Work out the finished part from the listing and answer in its coordinate system (mm). Round coordinates to 2 decimals unless told otherwise and drop trailing zeros. Order: outer loops, then holes, each group sorted by start corner. A loop starts at its lowest first (then second) coordinate and runs counter-clockwise, first axis right, second up. Notation, with made-up numbers: (-19, 56.25) -> (23, 56.25) arc R15 ccw to (23, 83.25) -> close; hole circle Ø3 at (83.25, -32). An arc over 180 degrees is marked (long way). Use a Markdown table: item, result. Add a question column.
Item 1: A cutting plane is placed at A-A, the plane z = 869. Determine the outline of the cut face in (x, y) (3 decimals).
Item 2: Find the intervals of material crossed by L1, parallel to X at y = 4.25, z = 679.5 (3 decimals); L2, parallel to Y at x = 11.5, z = 929 (3 decimals), in increasing order. Write a range as [from, to].
Item 3: Flat-ended cylindrical pins translate along their axes: P1, Ø4.5, axis at x = 11.11, z = 881.06, coming from the -Y side (1 decimal); P2, Ø7.5, axis at x = 15.5, z = 297, coming from the +Y side (3 decimals); P3, Ø4.5, axis at y = 7.94, z = 1136.02, coming from the -X side (3 decimals). Find the tip coordinate at first contact, or state that the pin passes through.
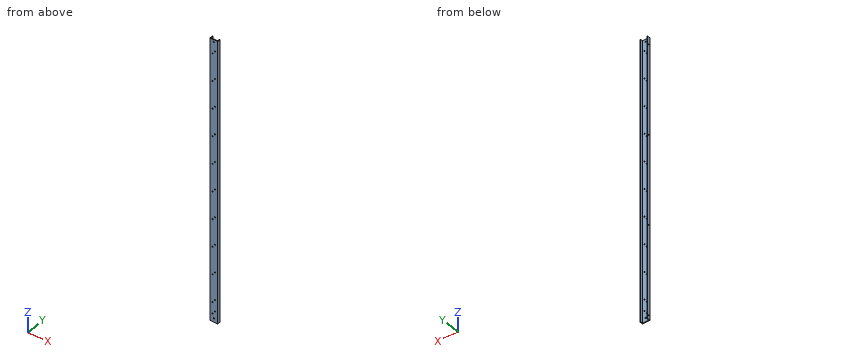
from build123d import *

# Parameters (mm, degrees)
BOSS_EXTRUDE1_DEPTH = 1168.4
CUT_EXTRUDE1_REACH  = 1170.87
SKETCH3_R           = 2.413
CUT_EXTRUDE2_REACH  = 1170.87
SKETCH4_R           = 2.413
LPATTERN1_COUNT     = 10
LPATTERN1_PITCH     = 114.3
CUT_EXTRUDE3_REACH  = 1170.9
SKETCH5_R           = 2.413
CUT_EXTRUDE4_REACH  = 1170.9
SKETCH6_R           = 2.413
CUT_EXTRUDE5_REACH  = 1170.87
SKETCH7_R           = 2.413


with BuildPart() as part:
    # Sketch1 → Boss-Extrude1 (new body)
    with BuildSketch(Plane.XY):
        Polygon((3.175, 3.175), (3.175, 12.7), (0, 12.7), (0, 0), (31.75, 0), (31.75, 12.7), (28.575, 12.7), (28.575, 3.175), align=None)
    extrude(amount=BOSS_EXTRUDE1_DEPTH)

    # Sketch3 → Cut-Extrude1 (cut, up to next)
    with BuildSketch(Plane(origin=(0, 3.175, 0), x_dir=(1, 0, 0), z_dir=(0, 1, 0)), mode=Mode.PRIVATE) as cut_extrude1_sk1:
        with Locations(Location((11.1125, -1109.6625, 0), (0, 0, 270))):
            Circle(SKETCH3_R)
    cut_extrude1_tool1 = extrude(cut_extrude1_sk1.sketch, amount=-CUT_EXTRUDE1_REACH, mode=Mode.PRIVATE) & part.part
    # Sketch3 → Cut-Extrude1 (cut, up to next)
    with BuildSketch(Plane(origin=(0, 3.175, 0), x_dir=(1, 0, 0), z_dir=(0, 1, 0)), mode=Mode.PRIVATE) as cut_extrude1_sk2:
        with Locations(Location((20.6375, -1122.3625, 0), (0, 0, 270))):
            Circle(SKETCH3_R)
    cut_extrude1_tool2 = extrude(cut_extrude1_sk2.sketch, amount=-CUT_EXTRUDE1_REACH, mode=Mode.PRIVATE) & part.part
    cut_extrude1_1 = cut_extrude1_tool1.solids().sort_by_distance((11.1125, 3.175, 1109.6625))[0]
    add(cut_extrude1_1, mode=Mode.SUBTRACT)
    cut_extrude1_2 = cut_extrude1_tool2.solids().sort_by_distance((20.6375, 3.175, 1122.3625))[0]
    add(cut_extrude1_2, mode=Mode.SUBTRACT)
    cut_extrude1 = cut_extrude1_1 + cut_extrude1_2  # Cut-Extrude1 as one shape, for the pattern or mirror that repeats it

    # Sketch4 → Cut-Extrude2 (cut, up to next)
    with BuildSketch(Plane(origin=(0, 3.175, 0), x_dir=(1, 0, 0), z_dir=(0, 1, 0)), mode=Mode.PRIVATE) as cut_extrude2_sk1:
        with Locations(Location((15.875, -1158.875, 0), (0, 0, 270))):
            Circle(SKETCH4_R)
    cut_extrude2_tool1 = extrude(cut_extrude2_sk1.sketch, amount=-CUT_EXTRUDE2_REACH, mode=Mode.PRIVATE) & part.part
    add(cut_extrude2_tool1.solids().sort_by_distance((15.875, 3.175, 1158.875))[0], mode=Mode.SUBTRACT)

    # LPattern1: Cut-Extrude1 ×10
    with Locations(*[(0, 0, -i * LPATTERN1_PITCH) for i in range(1, LPATTERN1_COUNT)]):
        add(cut_extrude1, mode=Mode.SUBTRACT)

    # Sketch5 → Cut-Extrude3 (cut, up to next)
    with BuildSketch(Plane.ZY, mode=Mode.PRIVATE) as cut_extrude3_sk1:
        with Locations((15.875, 7.9375)):
            Circle(SKETCH5_R)
    cut_extrude3_tool1 = extrude(cut_extrude3_sk1.sketch, amount=-CUT_EXTRUDE3_REACH, mode=Mode.PRIVATE) & part.part
    # Sketch5 → Cut-Extrude3 (cut, up to next)
    with BuildSketch(Plane.ZY, mode=Mode.PRIVATE) as cut_extrude3_sk2:
        with Locations((389.255, 7.9375)):
            Circle(SKETCH5_R)
    cut_extrude3_tool2 = extrude(cut_extrude3_sk2.sketch, amount=-CUT_EXTRUDE3_REACH, mode=Mode.PRIVATE) & part.part
    # Sketch5 → Cut-Extrude3 (cut, up to next)
    with BuildSketch(Plane.ZY, mode=Mode.PRIVATE) as cut_extrude3_sk3:
        with Locations((762.635, 7.9375)):
            Circle(SKETCH5_R)
    cut_extrude3_tool3 = extrude(cut_extrude3_sk3.sketch, amount=-CUT_EXTRUDE3_REACH, mode=Mode.PRIVATE) & part.part
    # Sketch5 → Cut-Extrude3 (cut, up to next)
    with BuildSketch(Plane.ZY, mode=Mode.PRIVATE) as cut_extrude3_sk4:
        with Locations((1136.015, 7.9375)):
            Circle(SKETCH5_R)
    cut_extrude3_tool4 = extrude(cut_extrude3_sk4.sketch, amount=-CUT_EXTRUDE3_REACH, mode=Mode.PRIVATE) & part.part
    add(cut_extrude3_tool1.solids().sort_by_distance((0, 7.9375, 15.875))[0], mode=Mode.SUBTRACT)
    add(cut_extrude3_tool2.solids().sort_by_distance((0, 7.9375, 389.255))[0], mode=Mode.SUBTRACT)
    add(cut_extrude3_tool3.solids().sort_by_distance((0, 7.9375, 762.635))[0], mode=Mode.SUBTRACT)
    add(cut_extrude3_tool4.solids().sort_by_distance((0, 7.9375, 1136.015))[0], mode=Mode.SUBTRACT)

    # Sketch6 → Cut-Extrude4 (cut, up to next)
    with BuildSketch(Plane.XZ, mode=Mode.PRIVATE) as cut_extrude4_sk1:
        with Locations(Location((11.1125, 33.3375, 0), (0, 0, 270))):
            Circle(SKETCH6_R)
    cut_extrude4_tool1 = extrude(cut_extrude4_sk1.sketch, amount=-CUT_EXTRUDE4_REACH, mode=Mode.PRIVATE) & part.part
    # Sketch6 → Cut-Extrude4 (cut, up to next)
    with BuildSketch(Plane.XZ, mode=Mode.PRIVATE) as cut_extrude4_sk2:
        with Locations(Location((20.6375, 46.0375, 0), (0, 0, 270))):
            Circle(SKETCH6_R)
    cut_extrude4_tool2 = extrude(cut_extrude4_sk2.sketch, amount=-CUT_EXTRUDE4_REACH, mode=Mode.PRIVATE) & part.part
    add(cut_extrude4_tool1.solids().sort_by_distance((11.1125, 0, 33.3375))[0], mode=Mode.SUBTRACT)
    add(cut_extrude4_tool2.solids().sort_by_distance((20.6375, 0, 46.0375))[0], mode=Mode.SUBTRACT)

    # Sketch7 → Cut-Extrude5 (cut, up to next)
    with BuildSketch(Plane(origin=(0, 3.175, 0), x_dir=(1, 0, 0), z_dir=(0, 1, 0)), mode=Mode.PRIVATE) as cut_extrude5_sk1:
        with Locations(Location((15.875, -15.875, 0), (0, 0, 270))):
            Circle(SKETCH7_R)
    cut_extrude5_tool1 = extrude(cut_extrude5_sk1.sketch, amount=-CUT_EXTRUDE5_REACH, mode=Mode.PRIVATE) & part.part
    add(cut_extrude5_tool1.solids().sort_by_distance((15.875, 3.175, 15.875))[0], mode=Mode.SUBTRACT)


solid = part.part
Reported:
| question | item | result |
|---|---|---|
| 1 | outline | (0, 0) -> (31.75, 0) -> (31.75, 12.7) -> (28.575, 12.7) -> (28.575, 3.175) -> (3.175, 3.175) -> (3.175, 12.7) -> (0, 12.7) -> close |
| 2 | L1 | [0, 3.175], [28.575, 31.75] |
| 2 | L2 | [0, 3.175] |
| 3 | P1 | through |
| 3 | P2 | y = 3.175 |
| 3 | P3 | x = 28.575 |
